CAD build for the part. Positions are in the model's coordinates, mm. A direction names the side the tool comes from. Round coordinates to 2 decimals unless told otherwise and drop trailing zeros. Loops run counter-clockwise (first coordinate to the right, second up) from the corner with the lowest first, then second, coordinate; pieces in that order, holes last. Notation, with made-up numbers: M 73,16 L 102,16 A20 cw 102,50 Z; hole C -15,48 d3. An arc over 180 degrees is marked long. Put each result on its own line as item: value. Start each with the question number.
from build123d import *

# Parameters (mm, degrees)
CROQUIS1_R              = 14
SALIENTE_EXTRUIR1_DEPTH = 85
CROQUIS2_OUTSIDE_W      = 48.754
CROQUIS2_OUTSIDE_H      = 48.754
CROQUIS2_OUTSIDE_R      = 10.65
CORTAR_EXTRUIR2_DEPTH   = 18
CORTAR_EXTRUIR3_START   = -55.7
CROQUIS5_R              = 14
CORTAR_EXTRUIR3_DEPTH   = 55.7
CROQUIS6_R              = 8.35
SALIENTE_EXTRUIR2_DEPTH = 73.1
CROQUIS7_OUTSIDE_W      = 51.958
CROQUIS7_OUTSIDE_H      = 51.958
CROQUIS7_OUTSIDE_R      = 10.5
CORTAR_EXTRUIR5_DEPTH   = 18


with BuildPart() as part:
    # Croquis1 → Saliente-Extruir1 (new body)
    with BuildSketch(Plane.XY):
        Circle(CROQUIS1_R)
    extrude(amount=SALIENTE_EXTRUIR1_DEPTH)

    # Croquis2 outside → Cortar-Extruir2 (cut)
    with BuildSketch(Plane(origin=(0, 0, 0), x_dir=(-1, 0, 0), z_dir=(0, 0, -1))):
        Rectangle(CROQUIS2_OUTSIDE_W, CROQUIS2_OUTSIDE_H)
        Circle(CROQUIS2_OUTSIDE_R, mode=Mode.SUBTRACT)
    extrude(amount=-CORTAR_EXTRUIR2_DEPTH, mode=Mode.SUBTRACT)

    # Croquis5 → Cortar-Extruir3 (cut)
    with BuildSketch(Plane.XY.offset(85).offset(CORTAR_EXTRUIR3_START)):
        with Locations(Location((0, 0, 0), (0, 0, 180))):
            Circle(CROQUIS5_R)
    extrude(amount=CORTAR_EXTRUIR3_DEPTH, mode=Mode.SUBTRACT)

    # Croquis6 → Saliente-Extruir2 (add)
    with BuildSketch(Plane.XY.offset(29.3)):
        Circle(CROQUIS6_R)
    extrude(amount=SALIENTE_EXTRUIR2_DEPTH)

    # Croquis7 outside → Cortar-Extruir5 (cut)
    with BuildSketch(Plane(origin=(0, 0, 0), x_dir=(-1, 0, 0), z_dir=(0, 0, -1))):
        Rectangle(CROQUIS7_OUTSIDE_W, CROQUIS7_OUTSIDE_H)
        Circle(CROQUIS7_OUTSIDE_R, mode=Mode.SUBTRACT)
    extrude(amount=-CORTAR_EXTRUIR5_DEPTH, mode=Mode.SUBTRACT)


solid = part.part
(1) Drill centre lines: line 1 along Y through (x, z) = (0.5, 55.5); line 2 along Z through (x, y) = (10, 6.5); line 3 along Z through (x, y) = (-3.5, 9.5). Where is each one in solid material? Low to high.
(2) Flat gauge pins, fed straight in: pin 1 Ø8 at (x, y) = (-8.5, -11) entering from +Z; pin 2 Ø1 at (y, z) = (6, 88) entering from -X; pin 3 Ø5 at (y, z) = (-4.5, 42) entering from -X. Where does each tip first touch, or does it go through?
(3) Tool access for faces 1 (the cylindrical face through (7.964, 2.508, 65.338)), 2 (the flat face through (0, 0, 102.4)), 3 (the flat face through (-5.1, 9.4, 18)): list every direction of +Z, -Z, +X, -X, +Y, -Y with a clear straight run to the whole face (end or side of a thin tool).
(4) Cut at A-A on x = 0. List the corners of the cut face in (y, z).
(5) Cut at C-C on z = 13. List the corners of the cut face in (x, y).
(6) Cut at D-D on x = 9.5. List the corners of the cut face in (y, z), and give its area (3 significant figures).
Taken from the geometry:
1. line 1: -8.34 to 8.34
1. line 2: 18 to 29.3
1. line 3: 0 to 29.3
2. pin 1: z = 29.3
2. pin 2: x = -6.28
2. pin 3: x = -8.11
3. face 1: +Z
3. face 2: +Z, +X, -X, +Y, -Y
3. face 3: -Z
4. outline: M -14,18 L -10.5,18 L -10.5,0 L 10.5,0 L 10.5,18 L 14,18 L 14,29.3 L 8.35,29.3 L 8.35,102.4 L -8.35,102.4 L -8.35,29.3 L -14,29.3 Z
5. outline: C 0,0 d21
6. outline: M -10.28,18 L -4.47,18 L -4.47,0 L 4.47,0 L 4.47,18 L 10.28,18 L 10.28,29.3 L -10.28,29.3 Z
6. area: 393 mm2
